from build123d import *
from build123d.topology import SkipClean

# Parameters (mm, degrees)
SKETCH_1_R          = 5.5
EXTRUDE_1_DEPTH     = 25
EXTRUDE_2_DEPTH     = 38
SKETCH_3_R          = 2.5
EXTRUDE_4_DEPTH     = 6
CHAMFER_1_SIZE      = 0.25
CUT_EXTRUDE_1_DEPTH = 15
SKETCH_6_R          = 3
CUT_EXTRUDE_2_DEPTH = 3
M3X0_5_1_D          = 2.5
M3X0_5_1_DEPTH      = 3


with BuildPart() as part:
    # Sketch 1 → Extrude 1 (new body)
    with BuildSketch(Plane(origin=(0, 0, 0), x_dir=(1, 0, 0), z_dir=(0, 1, 0))):
        with Locations(Location((0, 0, 0), (0, 0, 270))):  # turned: the seam where the file's is
            Circle(SKETCH_1_R)
    extrude(amount=EXTRUDE_1_DEPTH)

    # Sketch 2 → Extrude 2 (add)
    with BuildSketch(Plane(origin=(0, 25, 0), x_dir=(1, 0, 0), z_dir=(0, 1, 0))):
        Polygon((0, -4.67653718), (4.05, -2.33826859), (4.05, 2.33826859), (0, 4.67653718), (-4.05, 2.33826859), (-4.05, -2.33826859), align=None)
    extrude(amount=EXTRUDE_2_DEPTH)

    # Sketch 3 → Extrude 4 (add)
    with BuildSketch(Plane(origin=(0, 63, 0), x_dir=(1, 0, 0), z_dir=(0, 1, 0))):
        with Locations(Location((0, 0, 0), (0, 0, 270))):  # turned: the seam where the file's is
            Circle(SKETCH_3_R)
    extrude(amount=EXTRUDE_4_DEPTH)

    # Chamfer 1
    chamfer_1_edges = [part.edges().sort_by_distance(p)[0] for p in [
        (0, 69, -2.5),
    ]]
    chamfer(chamfer_1_edges, length=CHAMFER_1_SIZE)

    # Sketch 5 → Cut-Extrude 1 (cut)
    with BuildSketch(Plane.XZ):
        with BuildLine():
            Line((2.5, 1.658312395), (2.5, -1.658312395))
            ThreePointArc((2.5, -1.658312395), (-3, 0), (2.5, 1.658312395))
        make_face()
    extrude(amount=-CUT_EXTRUDE_1_DEPTH, mode=Mode.SUBTRACT)

    # Sketch 6 → Cut-Extrude 2 (cut)
    with SkipClean():  # keep this step's faces unmerged: merging them makes the solid invalid here
        with BuildSketch(Plane.XZ):
            with Locations(Location((0, 0, 0), (0, 0, 270))):  # turned: the seam where the file's is
                Circle(SKETCH_6_R)
        extrude(amount=-CUT_EXTRUDE_2_DEPTH, mode=Mode.SUBTRACT)

    # M3x0.5 _1
    with Locations(Plane.ZY.offset(-2.5)):
        with Locations((0, 9)):
            Hole(M3X0_5_1_D / 2, depth=M3X0_5_1_DEPTH)


solid = part.part
Model file for the job. Use its own axes, mm. A direction names the side the tool comes from. Coordinates: 2 decimals unless noted, no trailing zeros. Loops run counter-clockwise (first coordinate to the right, second up) from the corner with the lowest first, then second, coordinate; pieces in that order, holes last. Notation, with made-up numbers: (31, -13.5) -> (57, -13.5) arc R22 ccw to (57, 16.5) -> close; hole circle Ø10 at (67, 3.25). An arc over 180 degrees is marked (long way). Use one line per item in the form item = value. Start each with the question number.
(1) Cut at C-C on y = 9. Give the cut face in (x, z), and give its area (3 significant figures).
(2) Tool access for faces 1 (the flat face through (2, 43.73, 3.52)), 2 (the flat face through (-2, 43.73, -3.52)), 3 (the flat face through (2.5, 7.6, 0)), 4 (the cylindrical face through (-2.44, 65.83, -0.54)), 5 (the flat face through (4.05, 44, 0)): list every direction of +Z, -Z, +X, -X, +Y, -Y with a clear straight run to the whole face (end or side of a thin tool).
(3) Probe probe 1 along Y at (x, z) = (3.4, 0); probe 2 along Y at (x, z) = (4.1, 0); probe 3 along Y at (x, z) = (-2.5, -3). List the from-to ranges inside material, lowest first. Write a range as from..to.
(4) Cut at B-B on y = 30. Give the cut face in (x, z).
(5) Cut at A-A on z = 0. Give the cut face in (x, y), and give its area (3 significant figures).
(6) Pull direction X, two halves, no side cores. Call faces 6 (the flat face through (0, 15, 0)), 7 (the flat face through (-2, 63, 2)), 8 (the cylindrical face through (-5.37, 12.32, -1.19)), 9 (the flat face through (-4.05, 44, 0)): pulls with the +X half, pulls with the -X half, needs draft (parallel to the pull), parting line crosses it, or undercut.
(7) Flat gauge pins, fed straight in: pin 1 (2 mm diameter, centred on y = 29.5, z = 2.5, fed in from +X); pin 2 (1.7 mm diameter, centred on y = 6, z = 0.5, fed in from -X); pin 3 (5 mm diameter, centred on x = -4, y = 17, fed in from -Z); pin 4 (1.4 mm diameter, centred on y = 43, z = 0, fed in from -X). Where does each tip first touch, or does it go through?
Values:
q1.outline = (2.5, -1.66) arc R3 cw (long way) to (2.5, 1.66) -> (2.5, 1.25) -> (5.36, 1.25) arc R5.5 ccw (long way) to (5.36, -1.25) -> (2.5, -1.25) -> close
q1.area = 60.5 mm2
q2.face_1 = +Z, +X, +Y
q2.face_2 = -Z, -X, +Y
q2.face_3 = -Y
q2.face_4 = +Y
q2.face_5 = +Z, -Z, +X, +Y
q3.probe_1 = 0..7.75, 10.25..63
q3.probe_2 = 0..7.75, 10.25..25
q3.probe_3 = 0..63
q4.outline = (-4.05, -2.34) -> (0, -4.68) -> (4.05, -2.34) -> (4.05, 2.34) -> (0, 4.68) -> (-4.05, 2.34) -> close
q5.outline = (-5.5, 0) -> (-3, 0) -> (-3, 15) -> (2.5, 15) -> (2.5, 10.25) -> (5.5, 10.25) -> (5.5, 25) -> (4.05, 25) -> (4.05, 63) -> (2.5, 63) -> (2.5, 68.75) -> (2.25, 69) -> (-2.25, 69) -> (-2.5, 68.75) -> (-2.5, 63) -> (-4.05, 63) -> (-4.05, 25) -> (-5.5, 25) -> close; (2.5, 3) -> (3, 3) -> (3, 0) -> (5.5, 0) -> (5.5, 7.75) -> (2.5, 7.75) -> close
q5.area = 521 mm2
q6.face_6 = undercut
q6.face_7 = needs draft
q6.face_8 = parting line crosses it
q6.face_9 = pulls with the -X half
q7.pin_1 = 4.05
q7.pin_2 = -5.5
q7.pin_3 = -5.29
q7.pin_4 = -4.05
